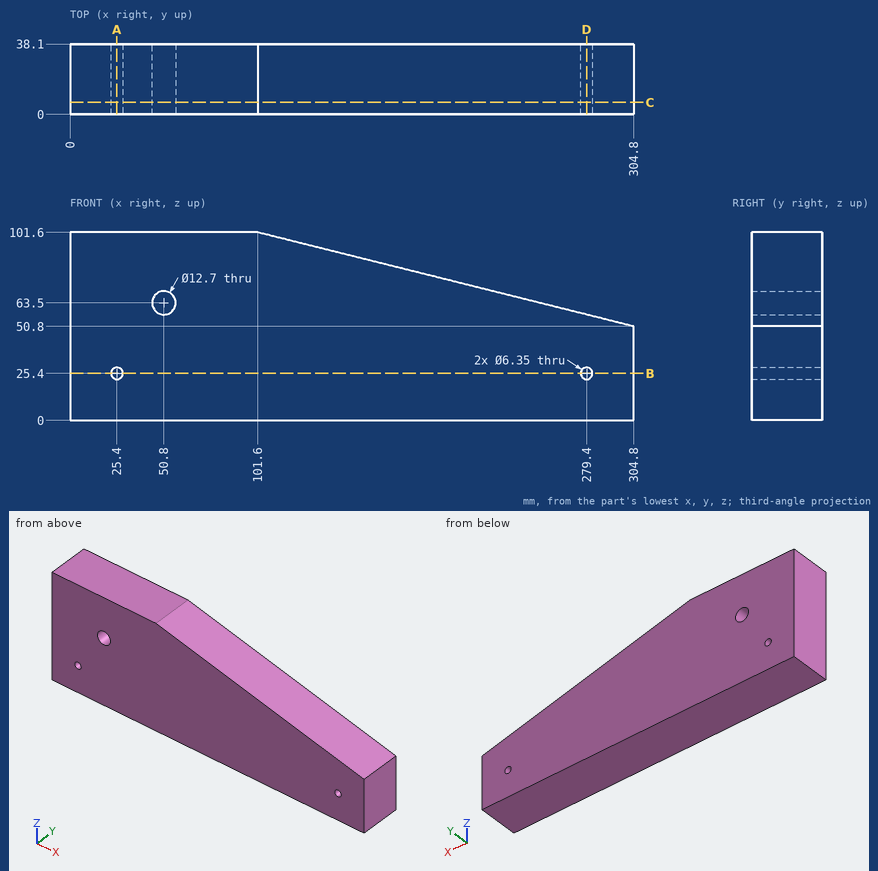
For this review, use the dimensioned drawing (mm, ordinates from the lowest corner) and the shaded views. Coordinates: 2 decimals unless noted, no trailing zeros. Write each loop counter-clockwise with the first axis right and the second up, starting at its lowest first coordinate (ties: lowest second). Pieces come first, ordered by that corner, then holes. Notation, with made-up numbers: (79, 48.25) - (90, 48.25) arc R22 ccw to (90, 79.25) - close; hole circle Ø5 at (-34, 40). An arc over 180 degrees is marked (long way). Answer in a Markdown table with one row per item. Add a question column.
Q1. To check wall thickness, follow line 1 along X through (y, z) = (25, 25); line 2 along X through (y, z) = (12, 25.5); line 3 along Z through (x, y) = (279.4, 15) (3 decimals). State the ranges of each line that lie inside material, in increasing order. Write a range as from..to.
Q2. Consider section B-B on z = 25.4. Give the boundary of the cut face in (x, y) (3 decimals).
Q3. Consider section A-A on x = 25.4. Give the boundary of the cut face in (y, z) (3 decimals), then the cut area to 3 significant figures.
Q4. Clearance check with flat-ended pins moving along their axes: pin 1 (3 mm diameter, centred on x = 173.5, y = 31.5, fed in from +Z); pin 2 (4 mm diameter, centred on x = 180, y = 24, fed in from +Z); pin 3 (6 mm diameter, centred on x = 175.5, y = 16, fed in from +Z) (3 decimals). State where each tip first meets the part, or that it passes through.
Q5. Consider section C-C on y = 6.5. Give the boundary of the cut face in (x, z) (3 decimals).
Q6. Consider section D-D on x = 279.4. Give the boundary of the cut face in (y, z) (3 decimals), then the cut area to 3 significant figures.
Answers below:
| question | item | result |
|---|---|---|
| 1 | line 1 | 0..22.25, 28.55..276.25, 282.55..304.8 |
| 1 | line 2 | 0..22.23, 28.57..276.23, 282.57..304.8 |
| 1 | line 3 | 0..22.225, 28.575..57.15 |
| 2 | outline | (0, 0) - (22.225, 0) - (22.225, 38.1) - (0, 38.1) - close; (28.575, 0) - (276.225, 0) - (276.225, 38.1) - (28.575, 38.1) - close; (282.575, 0) - (304.8, 0) - (304.8, 38.1) - (282.575, 38.1) - close |
| 3 | outline | (0, 0) - (38.1, 0) - (38.1, 22.225) - (0, 22.225) - close; (0, 28.575) - (38.1, 28.575) - (38.1, 101.6) - (0, 101.6) - close |
| 3 | area | 3,630 mm² |
| 4 | pin 1 | z = 84 |
| 4 | pin 2 | z = 82.5 |
| 4 | pin 3 | z = 83.875 |
| 5 | outline | (0, 0) - (304.8, 0) - (304.8, 50.8) - (101.6, 101.6) - (0, 101.6) - close; hole circle Ø6.35 at (25.4, 25.4); hole circle Ø12.7 at (50.8, 63.5); hole circle Ø6.35 at (279.4, 25.4) |
| 6 | outline | (0, 0) - (38.1, 0) - (38.1, 22.225) - (0, 22.225) - close; (0, 28.575) - (38.1, 28.575) - (38.1, 57.15) - (0, 57.15) - close |
| 6 | area | 1,940 mm² |
